Input: dimensioned drawing with shaded views. Units: mm. Origin: part minimum x, y, z. Coordinates: 2 decimals unless noted, no trailing zeros. Loops run counter-clockwise (first coordinate to the right, second up) from the corner with the lowest first, then second, coordinate; pieces in that order, holes last.
Item 1: Ray query, line 1 along Z through (x, y) = (36, 3.5); line 2 along X through (y, z) = (6.25, 9.5) (1 decimal); line 3 along X through (y, z) = (3.5, 11) (1 decimal). Return the intervals inside material, ascending.
Item 2: Section B-B on x = 22.5. Return loops of the section in (y, z), and give its area (3 significant figures).
Item 3: Section A-A on z = 22.5. Return loops of the section in (x, y), and give its area (3 significant figures).
Item 4: Section C-C on x = 35.5. Return loops of the section in (y, z) (1 decimal).
Item 5: Section D-D on z = 29. Return loops of the section in (x, y).
Item 6: Pull-direction query (Z, two-part tool) for the marked faces 1, 2 and 3; classes: released by +Z, released by -Z, zero draft, split by the parting line, or undercut.
Item 7: Contact query for flat-ended pins moving along their axis: P1, Ø0.6, axis at y = 1, z = 21, coming from the -X side; P2, Ø4, axis at x = 28.5, y = 1.5, coming from the -Z side; P3, Ø4, axis at y = 4.5, z = 14.5, coming from the -X side (1 decimal). Output: stop coordinate, or through.
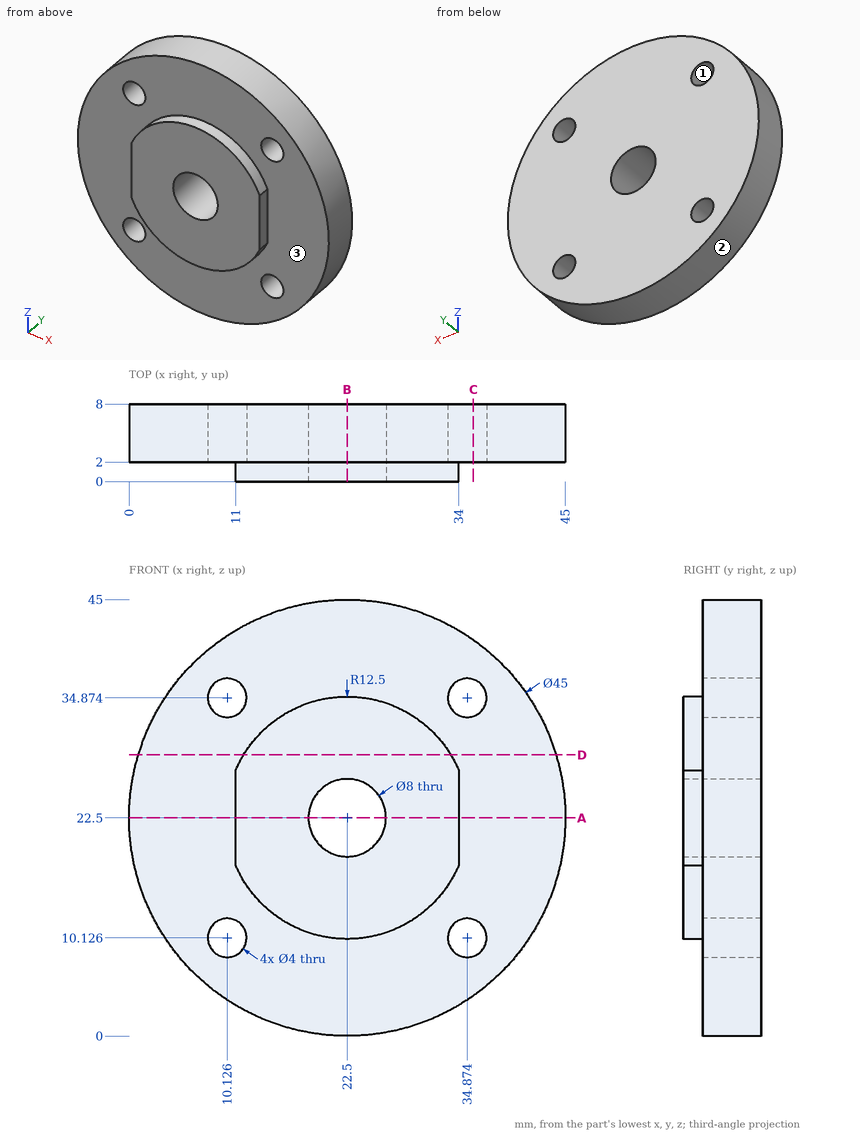
Results found:
1. line 1: z = 4.5 to 8.47, 11.78 to 33.22, 36.53 to 40.5
1. line 2: x = 4.1 to 8.2, 12 to 33, 36.8 to 40.9
1. line 3: x = 3.2 to 8.3, 11.9 to 33.1, 36.7 to 41.8
2. outline: (0, 10) - (2, 10) - (2, 0) - (8, 0) - (8, 18.5) - (0, 18.5) - close; (0, 26.5) - (8, 26.5) - (8, 45) - (2, 45) - (2, 35) - (0, 35) - close
2. area: 256 mm2
3. outline: (0, 2) - (11, 2) - (11, 0) - (18.5, 0) - (18.5, 8) - (0, 8) - close; (26.5, 0) - (34, 0) - (34, 2) - (45, 2) - (45, 8) - (26.5, 8) - close
3. area: 252 mm2
4. outline: (2, 4.1) - (8, 4.1) - (8, 8.2) - (2, 8.2) - close; (2, 12) - (8, 12) - (8, 33) - (2, 33) - close; (2, 36.8) - (8, 36.8) - (8, 40.9) - (2, 40.9) - close
5. outline: (0.96, 2) - (11.82, 2) - (11.82, 0) - (33.18, 0) - (33.18, 2) - (44.04, 2) - (44.04, 8) - (0.96, 8) - close
6. face 1: undercut
6. face 2: split by the parting line
6. face 3: zero draft
7. P1: stops at x = 11
7. P2: stops at z = 0.37
7. P3: stops at x = 0.8
